Job drawing, mm, ordinate dimensions from the low corner. One solid piece. Coordinates: 2 decimals unless noted, no trailing zeros. Loops run counter-clockwise (first coordinate to the right, second up) from the corner with the lowest first, then second, coordinate; pieces in that order, holes last. Notation, with made-up numbers: (-3, 73.5) -> (26, 73.5) arc R24 ccw to (26, 88.5) -> close; hole circle Ø7 at (-26, 18.25). An arc over 180 degrees is marked (long way). Answer as CSV lines item,"result". Start each with the question number.
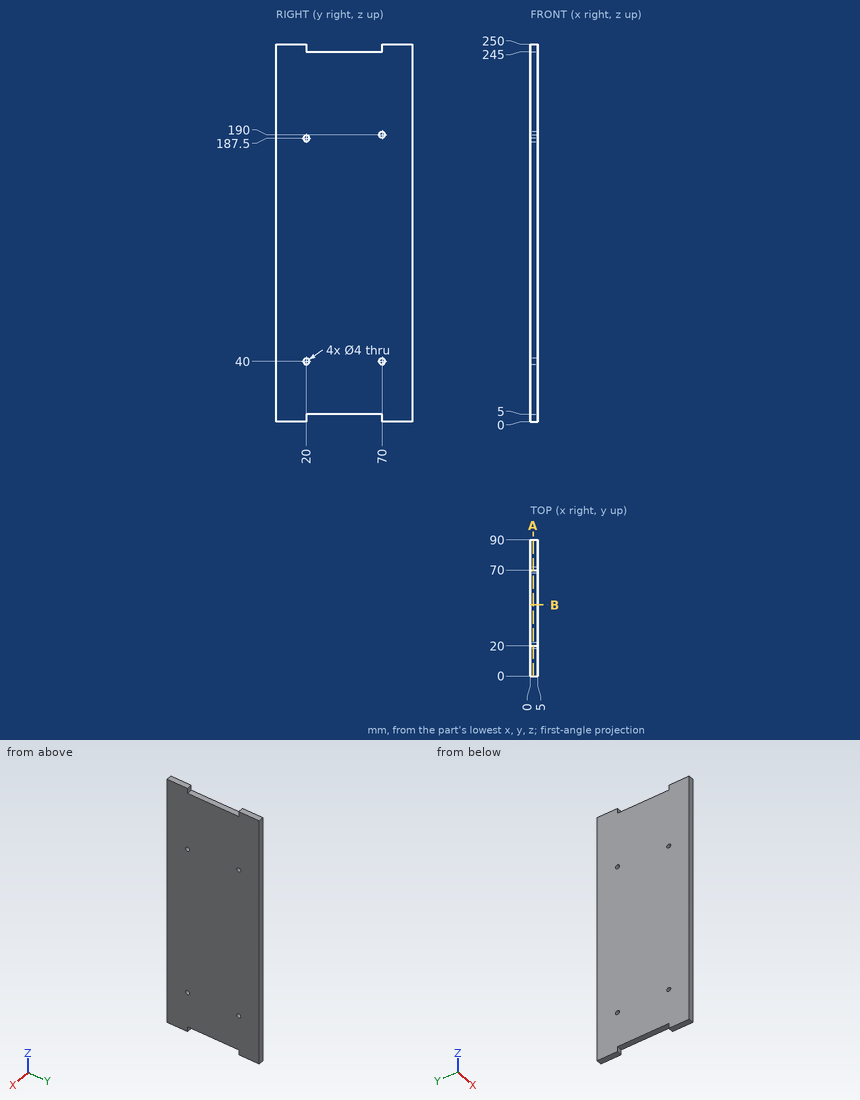
Q1. Saw through at B-B (y = 47). List the corners of the cut face in (x, z).
Q2. Probe probe 1 along Y at (x, z) = (1.25, 40); probe 2 along Y at (x, z) = (1.2, 190); probe 3 along Z at (x, y) = (2.3, 23). List the from-to ranges inside material, lowest first. Write a range as from..to.
Q3. Saw through at A-A (x = 1.95). List the corners of the cut face in (y, z).
Q4. Pin check, flat tip, straight feed: pin 1 Ø2.5 at (x, y) = (2, 56) entering from +Z. Stop position of the tip, or through.
Ans:
1,outline,"(0, 5) -> (5, 5) -> (5, 245) -> (0, 245) -> close"
2,probe 1,"y = 0..18, 22..68, 72..90"
2,probe 2,"y = 0..68, 72..90"
2,probe 3,"z = 5..245"
3,outline,"(0, 0) -> (20, 0) -> (20, 5) -> (70, 5) -> (70, 0) -> (90, 0) -> (90, 250) -> (70, 250) -> (70, 245) -> (20, 245) -> (20, 250) -> (0, 250) -> close; hole circle Ø4 at (20, 40); hole circle Ø4 at (20, 187.5); hole circle Ø4 at (70, 40); hole circle Ø4 at (70, 190)"
4,pin 1,"stops at z = 245"
